Check sheet for the modelled part. Datum: model origin and axes. Units: mm. A direction names the side the tool comes from. Coordinates: 2 decimals unless noted, no trailing zeros. Loops run counter-clockwise (first coordinate to the right, second up) from the corner with the lowest first, then second, coordinate; pieces in that order, holes last. Notation, with made-up numbers: M 15.5,30.5 L 42.5,30.5 A23 ccw 42.5,42.5 Z; hole C 39.5,-25.5 d5. An arc over 180 degrees is marked long. Return JSON: item names as keys, results as strings.
from build123d import *
from build123d.topology import SkipClean

# Parameters (mm, degrees)
SKETCH1_R           = 12
SKETCH1_R_2         = 7
SKETCH1_R_3         = 5.5
BOSS_EXTRUDE1_DEPTH = 2.9
SKETCH1_3_R         = 7
SKETCH1_3_R_2       = 5.5
BOSS_EXTRUDE2_DEPTH = 10
SKETCH2_R           = 5.5
CUT_EXTRUDE2_DEPTH  = 1
SKETCH3_R           = 5.5
CUT_EXTRUDE3_DEPTH  = 1
CUT_EXTRUDE4_START  = -2.5
SKETCH3_4_R         = 5.5
CUT_EXTRUDE4_DEPTH  = 2.5
CUT_EXTRUDE6_REACH  = 32.109
SKETCH5_R           = 1.55
CUT_EXTRUDE7_START  = -2.1
CUT_EXTRUDE7_DEPTH  = 2.1
SKETCH6_R           = 5.5
CUT_EXTRUDE8_DEPTH  = 2.1
FILLET1_R           = 10
SKETCH5_3_R         = 2.75
SKETCH5_3_R_2       = 1.55
CUT_EXTRUDE9_DEPTH  = 3


with BuildPart() as part:
    # Sketch1 → Boss-Extrude1 (new body)
    # profile 1 of 4: a face of its own
    with BuildSketch(Plane(origin=(0, 0, 0), x_dir=(1, 0, 0), z_dir=(0, 1, 0))):
        Circle(SKETCH1_R)
        Circle(SKETCH1_R_2, mode=Mode.SUBTRACT)
    # profile 2 of 4: a face of its own
    with BuildSketch(Plane(origin=(0, 0, 0), x_dir=(1, 0, 0), z_dir=(0, 1, 0))):
        with BuildLine():
            ThreePointArc((12, -2.94e-15), (11.769423369196444, -2.341083842286014), (11.086554407231223, -4.592201147108209))
            Line((11.086554407231223, -4.592201147108209), (17.959269151985882, 12))
            Line((17.959269151985882, 12), (17.959269151985882, 12.009999999999998))
            ThreePointArc((17.959269151985882, 12.009999999999998), (15.033265896039495, 19.07399674405361), (7.969269151985883, 21.999999999999996))
            Line((7.969269151985883, 21.999999999999996), (-7.969269151985883, 21.999999999999996))
            ThreePointArc((-7.969269151985883, 21.999999999999993), (-15.033265896039492, 19.07399674405361), (-17.959269151985882, 12.009999999999998))
            Line((-17.959269151985882, 12.009999999999998), (-17.959269151985882, 12))
            Line((-17.95926915198589, 12.000000000000014), (-11.086554257092926, -4.592201509574117))
            ThreePointArc((-11.08655425709292, -4.592201509574119), (-2.3410840346818973, 11.769423330926521), (12, 0))
        make_face()
    # profile 3 of 4: a face of its own
    with BuildSketch(Plane(origin=(0, 0, 0), x_dir=(1, 0, 0), z_dir=(0, 1, 0))):
        Circle(SKETCH1_R_2)
    # profile 4 of 4: a face of its own
    with BuildSketch(Plane(origin=(0, 0, 0), x_dir=(1, 0, 0), z_dir=(0, 1, 0))):
        Circle(SKETCH1_R_3)
    extrude(amount=BOSS_EXTRUDE1_DEPTH)

    # Sketch1<3> → Boss-Extrude2 (add)
    with BuildSketch(Plane(origin=(0, 0, 0), x_dir=(1, 0, 0), z_dir=(0, 1, 0))):
        with Locations(Location((0, 0, 0), (0, 0, 270))):
            Circle(SKETCH1_3_R)
        Circle(SKETCH1_3_R_2)
    extrude(amount=BOSS_EXTRUDE2_DEPTH)

    # Sketch2 → Cut-Extrude2 (cut)
    with SkipClean():  # the faces are left unmerged after this step: merging them gives an invalid solid
        with BuildSketch(Plane(origin=(0, 2.9, 0), x_dir=(1, 0, 0), z_dir=(0, 1, 0))):
            with BuildLine():
                ThreePointArc((-5.500000000000162, 4.330127018921988), (-1.9852e-13, 7), (5.499999999999917, 4.330127018922298))
                Line((5.5, 4.330127018922322), (5.5, 11.712224753227023))
                Line((5.5, 11.712224753227023), (-5.5, 11.712224753227023))
                Line((-5.5, 11.712224753227023), (-5.5, 4.330127018921939))
            make_face()
            with Locations(Location((0, 0, 0), (0, 0, 270))):
                Circle(SKETCH2_R)
        extrude(amount=CUT_EXTRUDE2_DEPTH, mode=Mode.SUBTRACT)

    # Sketch3 → Cut-Extrude3 (cut)
    with BuildSketch(Plane(origin=(0, 2.9, 0), x_dir=(1, 0, 0), z_dir=(0, 1, 0))):
        Circle(SKETCH3_R)
        with BuildLine():
            ThreePointArc((-5.5, 3.12e-15), (1.56e-15, 5.5), (5.5, 0))
            Line((5.5, 0), (6.1896702982743115, 13.159693230837554))
            Line((6.1896702982743115, 13.159693230837554), (-6.189670298274319, 13.159693230837554))
            Line((-6.1896702982743195, 13.159693230837554), (-5.5, 0))
        make_face()
    extrude(amount=CUT_EXTRUDE3_DEPTH, mode=Mode.SUBTRACT)

    # Sketch3<4> → Cut-Extrude4 (cut)
    with SkipClean():  # the faces are left unmerged after this step: merging them gives an invalid solid
        with BuildSketch(Plane(origin=(0, 2.9, 0), x_dir=(1, 0, 0), z_dir=(0, 1, 0)).offset(CUT_EXTRUDE4_START)):
            with Locations(Location((0, 0, 0), (0, 0, 180))):
                Circle(SKETCH3_4_R)
        extrude(amount=CUT_EXTRUDE4_DEPTH, mode=Mode.SUBTRACT)

    # Sketch5 → Cut-Extrude6 (cut, up to next)
    with BuildSketch(Plane(origin=(0, 10, 0), x_dir=(1, 0, 0), z_dir=(0, 1, 0)), mode=Mode.PRIVATE) as cut_extrude6_sk1:
        with Locations(Location((0, 0, 0), (0, 0, 270))):
            Circle(SKETCH5_R)
    cut_extrude6_tool1 = extrude(cut_extrude6_sk1.sketch, amount=-CUT_EXTRUDE6_REACH, mode=Mode.PRIVATE) & part.part
    add(cut_extrude6_tool1.solids().sort_by_distance((0, 10, 0))[0], mode=Mode.SUBTRACT)

    # Sketch3<5> → Cut-Extrude7 (cut)
    with BuildSketch(Plane(origin=(0, 2.9, 0), x_dir=(1, 0, 0), z_dir=(0, 1, 0)).offset(CUT_EXTRUDE7_START)):
        with BuildLine():
            ThreePointArc((-5.5, 3.12e-15), (1.56e-15, 5.5), (5.5, 0))
            Line((5.5, 0), (6.1896702982743115, 13.159693230837554))
            Line((6.1896702982743115, 13.159693230837554), (-6.189670298274319, 13.159693230837554))
            Line((-6.1896702982743195, 13.159693230837554), (-5.5, 0))
        make_face()
    extrude(amount=CUT_EXTRUDE7_DEPTH, mode=Mode.SUBTRACT)

    # Sketch6 → Cut-Extrude8 (cut)
    with BuildSketch(Plane(origin=(0, 2.9, 0), x_dir=(1, 0, 0), z_dir=(0, 1, 0))):
        with Locations((-4.34e-15, 13.159693230837554)):
            Circle(SKETCH6_R)
    extrude(amount=-CUT_EXTRUDE8_DEPTH, mode=Mode.SUBTRACT)

    # Fillet1
    # the kernel refuses this fillet: 10 mm, written as the material it takes off along each edge
    with BuildSketch(Plane(origin=(5.499999999999996, 8.022933245127838, -13.159693230837554), x_dir=(1, 0, 0), z_dir=(0, -1, 0))) as fillet1_piece_1:
        with BuildLine():
            CenterArc((8.924194649844473, -5.6738530738289406), FILLET1_R, 145.43190419239474, 13.095569895078825)
            ThreePointArc((-0.3817373823132515, -2.01330270361672), (-0.09627700574515341, -1.0245866490255686), (0, 0))
            Line((0, 0), (0.6896702982743177, 0))
        make_face()
    extrude(amount=7.222933245127838, mode=Mode.SUBTRACT)
    with BuildSketch(Plane(origin=(-5.500000000000004, 0.7999999999999998, -13.159693230837554), x_dir=(0.18628848164101172, 0, -0.9824950898645174), z_dir=(0, 1, 0))) as fillet1_piece_2:
        with BuildLine():
            CenterArc((3.9120581144612516, 9.824950898645172), FILLET1_R, 246.168167148658, 13.095569895078825)
            Line((-0.12847763269842533, 0.6775976816799091), (0, 0))
            ThreePointArc((0, 0), (1.0245866490255648, 0.09627700574515353), (2.0491732980511315, -1e-17))
        make_face()
    extrude(amount=7.222933245127831, mode=Mode.SUBTRACT)

    # Sketch5<3> → Cut-Extrude9 (cut)
    with BuildSketch(Plane(origin=(0, 10, 0), x_dir=(1, 0, 0), z_dir=(0, 1, 0))):
        with Locations(Location((0, 0, 0), (0, 0, 270))):
            Circle(SKETCH5_3_R)
        with Locations(Location((0, 0, 0), (0, 0, 270))):
            Circle(SKETCH5_3_R_2, mode=Mode.SUBTRACT)
    extrude(amount=-CUT_EXTRUDE9_DEPTH, mode=Mode.SUBTRACT)


solid = part.part
1) Scan lines: line 1 along X through (y, z) = (7.8, 0); line 2 along Y through (x, z) = (-1.5, -2.5); line 3 along X through (y, z) = (4.7, 0). Record each from-to range of solid material in increasing order. Write a range as [from, to].
Answers:
{"line 1": "[-7, -2.75], [2.75, 7]", "line 2": "[0, 0.4], [3.9, 10]", "line 3": "[-7, -1.55], [1.55, 7]"}
2) Section check C-C on z = -2. Record the cut outline in (x, y), then the cut area to 3 significant figures.
Answers:
{"outline": "M -13.82,0 L 13.82,0 L 13.82,2.9 L 6.71,2.9 L 6.71,10 L 1.89,10 L 1.89,7 L -1.89,7 L -1.89,10 L -6.71,10 L -6.71,2.9 L -13.82,2.9 Z; hole M -5.6,0.8 L -5.12,0.8 L -5.12,0.4 L 5.12,0.4 L 5.12,0.8 L 5.6,0.8 L 5.6,3.9 L -5.6,3.9 Z", "area": "125 mm²"}
3) Set-up check for faces 5 (the face through (0, 7, 2)), 6 (the face through (0, 3.9, -2)), 7 (the face through (-5.85, 1.98, -6.67)): record each of +Z, -Z, +X, -X, +Y, -Y from which the full face is reachable in a straight line by a thin tool's end or side.
Answers:
{"face 5": "+Y", "face 6": "-Z", "face 7": "none"}
4) Section check D-D on z = -17. Record the cut outline in (x, y).
Answers:
{"outline": "M -16.62,0 L 16.62,0 L 16.62,2.9 L 3.94,2.9 L 3.94,0.8 L -3.94,0.8 L -3.94,2.9 L -16.62,2.9 Z"}
5) Draft check along Y on faces 1 (the face through (0, 0.4, 0)), 2 (the face through (-2.681, 6.4, 6.466)), 3 (the face through (0, 0, -9)), 4 (the face through (5.84, 1.98, -6.49)). Enter one of: +Y half, -Y half, draft (parallel to the pull), parting line (faces both ways), or undercut.
Answers:
{"face 1": "undercut", "face 2": "draft", "face 3": "-Y half", "face 4": "undercut"}
6) Go/stop test with flat-tipped pins: pin 1 Ø1.5 at (y, z) = (3.5, -6) entering from -X; pin 2 Ø1.5 at (x, y) = (-11.5, 1.5) entering from -Z; pin 3 Ø2.5 at (x, z) = (0, 0) entering from +Y. Record where each tip stops, or that it passes through.
Answers:
{"pin 1": "x = -15.66", "pin 2": "z = -21.61", "pin 3": "y = 0.4"}
7) Section check B-B on x = 0. Record the cut outline in (y, z), then the cut area to 3 significant figures.
Answers:
{"outline": "M 0,-22 L 2.9,-22 L 2.9,-18.66 L 0.8,-18.66 L 0.8,-5.5 L 0.4,-5.5 L 0.4,5.5 L 3.9,5.5 L 3.9,1.55 L 7,1.55 L 7,2.75 L 10,2.75 L 10,7 L 2.9,7 L 2.9,12 L 0,12 Z; M 3.9,-7 L 10,-7 L 10,-2.75 L 7,-2.75 L 7,-1.55 L 3.9,-1.55 Z", "area": "104 mm²"}
